The model under review builds one solid part; all positions refer to its coordinate system, in mm. Face numbers are marked on the shaded views. A direction names the side the tool comes from. Give positions to 0.01 mm unless a question says otherwise; leave off trailing zeros. Loops run counter-clockwise (first coordinate to the right, second up) from the corner with the lowest first, then second, coordinate; pieces in that order, holes last. Notation, with made-up numbers: M 18,71.5 L 69,71.5 A16 ccw 69,99.5 Z; hole C -4,-5 d8. An arc over 180 degrees is marked long. One line per item, written item: value. Start each with the question number.
Q1. To check wall thickness, follow line 1 along Y through (x, z) = (0, 0.75); line 2 along Y through (x, z) = (0.5, -1.75); line 3 along Z through (x, y) = (-2, 1). State the ranges of each line that lie inside material, in increasing order. Write a range as from..to.
Q2. For the marked faces 4, 5 and 6, list the 3-axis set-ups (+Z, -Z, +X, -X, +Y, -Y) from which the entire face can be reached by the end or side of a thin tool; tool diameter is ignored.
Q3. We need section C-C on z = 2. Write out the cut boundary in (x, y).
Q4. For pin 1 (1.5 mm diameter, centred on y = 15, z = -0.5, fed in from -X); pin 2 (0.5 mm diameter, centred on x = -4, y = 6, fed in from +Z); pin 3 (0.7 mm diameter, centred on y = 11.5, z = 3.5, fed in from +X), all flat-tipped, find the tip position at first contact; note any pin that passes through.
Q5. We need section D-D on y = 2.25. Write out the cut boundary in (x, z), plus the area to 3 significant figures.
Q6. We need section A-A on x = 0. Write out the cut boundary in (y, z), plus the area to 3 significant figures.
Q7. Mouldability with a two-part tool opening along X and no side actions: class the marked faces 1, 2 and 3 as released by +X, released by -X, zero draft, split by the parting line, or undercut.
Q8. We need section B-B on y = 7. Write out the cut boundary in (x, z).
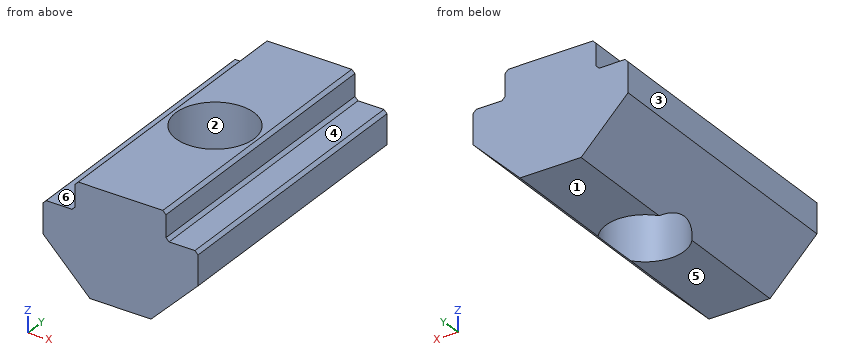
```python
from build123d import *

# Parameters (mm, degrees)
EXTRUDE_1_DEPTH    = 18
CHAMFER_1_SIZE     = 3
CHAMFER_2_SIZE     = 0.2
HOLE_WIZARD_M6_1_D = 5


with BuildPart() as part:
    # 草图1 → 凸台-拉伸1 (new body)
    with BuildSketch(Plane(origin=(0, 0, 0), x_dir=(1, 0, 0), z_dir=(0, 1, 0))):
        Polygon((2.9, -2.55), (4.95, -2.55), (4.95, 2.55), (-4.95, 2.55), (-4.95, -2.55), (-2.9, -2.55), (-2.9, -4.35), (2.9, -4.35), align=None)
    extrude(amount=EXTRUDE_1_DEPTH)

    # 倒角1
    chamfer_1_edges = [part.edges().sort_by_distance(p)[0] for p in [
        (-4.95, 9, -2.55),
        (4.95, 9, -2.55),
    ]]
    chamfer(chamfer_1_edges, length=CHAMFER_1_SIZE)

    # 倒角2
    chamfer_2_edges = [part.edges().sort_by_distance(p)[0] for p in [
        (4.95, 9, 2.55),
        (2.9, 9, 2.55),
        (2.9, 9, 4.35),
        (-2.9, 9, 4.35),
        (-2.9, 9, 2.55),
        (-4.95, 9, 2.55),
    ]]
    chamfer(chamfer_2_edges, length=CHAMFER_2_SIZE)

    # M6 螺纹孔1 (through all)
    with Locations(Plane.XY.offset(4.35)):
        with Locations((0, 9)):
            Hole(HOLE_WIZARD_M6_1_D / 2)


solid = part.part
```
Solved:
1. line 1: 0..6.5, 11.5..18
1. line 2: 0..6.55, 11.45..18
1. line 3: -2.5..4.35
2. face 4: +Z, +X, +Y, -Y
2. face 5: -Z, +X, -X, +Y, -Y
2. face 6: +Z, -X, +Y, -Y
3. outline: M -4.95,0 L 4.95,0 L 4.95,18 L -4.95,18 Z; hole C 0,9 d5
4. pin 1: x = -4.75
4. pin 2: z = 2.55
4. pin 3: x = 2.9
5. outline: M -4.95,0.45 L -1.95,-2.55 L 1.95,-2.55 L 4.95,0.45 L 4.95,2.35 L 4.75,2.55 L 3.1,2.55 L 2.9,2.75 L 2.9,4.15 L 2.7,4.35 L -2.7,4.35 L -2.9,4.15 L -2.9,2.75 L -3.1,2.55 L -4.75,2.55 L -4.95,2.35 Z
5. area: 51.9 mm2
6. outline: M 0,-2.55 L 6.5,-2.55 L 6.5,4.35 L 0,4.35 Z; M 11.5,-2.55 L 18,-2.55 L 18,4.35 L 11.5,4.35 Z
6. area: 89.7 mm2
7. face 1: zero draft
7. face 2: undercut
7. face 3: released by -X
8. outline: M -4.95,0.45 L -1.95,-2.55 L -1.5,-2.55 L -1.5,4.35 L -2.7,4.35 L -2.9,4.15 L -2.9,2.75 L -3.1,2.55 L -4.75,2.55 L -4.95,2.35 Z; M 1.5,-2.55 L 1.95,-2.55 L 4.95,0.45 L 4.95,2.35 L 4.75,2.55 L 3.1,2.55 L 2.9,2.75 L 2.9,4.15 L 2.7,4.35 L 1.5,4.35 Z
